from build123d import *

# Parameters (mm, degrees)
SKETCH1_W          = 25.4
SKETCH1_H          = 25.4
SKETCH1_W_2        = 19.05
SKETCH1_H_2        = 19.05
EXTRUDE1_DEPTH     = 558.8
SKETCH2_R          = 3.2639
CUT_EXTRUDE1_DEPTH = 26.4


with BuildPart() as part:
    # Sketch1 → Extrude1 (new body)
    with BuildSketch(Plane(origin=(0, 0, 0), x_dir=(0, 0, -1), z_dir=(1, 0, 0))):
        with Locations((12.7, 12.7)):
            Rectangle(SKETCH1_W, SKETCH1_H)
        with Locations((12.7, 12.7)):
            Rectangle(SKETCH1_W_2, SKETCH1_H_2, mode=Mode.SUBTRACT)
    extrude(amount=EXTRUDE1_DEPTH)

    # Sketch2 → Cut-Extrude1 (cut, through all)
    with BuildSketch(Plane(origin=(0, 25.4, 0), x_dir=(-1, 0, 0), z_dir=(0, 1, 0))):
        with Locations((-546.1, -12.7)):
            Circle(SKETCH2_R)
        with Locations((-368.3, -12.7)):
            Circle(SKETCH2_R)
        with Locations((-190.5, -12.7)):
            Circle(SKETCH2_R)
        with Locations((-12.7, -12.7)):
            Circle(SKETCH2_R)
    extrude(amount=-CUT_EXTRUDE1_DEPTH, mode=Mode.SUBTRACT)


solid = part.part
Model file for the job. Use its own axes, mm. A direction names the side the tool comes from. Coordinates: 2 decimals unless noted, no trailing zeros. Order: outer loops, then holes, each group sorted by start corner. A loop starts at its lowest first (then second) coordinate and runs counter-clockwise, first axis right, second up. Notation, with made-up numbers: M 83.5,21.5 L 122.5,21.5 A7 cw 122.5,25.5 Z; hole C -36,-2 d11. An arc over 180 degrees is marked long. Return JSON: item names as keys, results as strings.
1. Saw through at A-A (y = 16.75). Give the cut face in (x, z) (3 decimals), and give its area (3 significant figures).
Ans:
{"outline": "M 0,-25.4 L 558.8,-25.4 L 558.8,-22.225 L 0,-22.225 Z; M 0,-3.175 L 558.8,-3.175 L 558.8,0 L 0,0 Z", "area": "3,550 mm^2"}
2. Pull direction Z, two halves, no side cores. Call faces 1 (the face through (275, 13, -25.4)), 2 (the face through (275, 13, 0)), 3 (the face through (275, 13, -3.175)): +Z half, -Z half, draft (parallel to the pull), parting line (faces both ways), or undercut.
Ans:
{"face 1": "-Z half", "face 2": "+Z half", "face 3": "undercut"}
3. Flat gauge pin, fed straight in: pin 1 (5 mm diameter, centred on x = 368.3, z = -12.7, fed in from -Y). Where does the tip first touch, or does it go through?
Ans:
{"pin 1": "through"}
4. Drill centre lines: probe 1 along Y at (x, z) = (381.5, -13.75) (3 decimals); probe 2 along Z at (x, y) = (429, 21.25) (3 decimals); probe 3 along Z at (x, y) = (368.3, 1.85). Where is each one in solid material? Low to high.
Ans:
{"probe 1": "0 to 3.175, 22.225 to 25.4", "probe 2": "-25.4 to -22.225, -3.175 to 0", "probe 3": "-25.4 to -15.96, -9.44 to 0"}
5. Tool access for faces 4 (the face through (275, 0, -13)), 5 (the face through (275, 22.225, -13)): list every direction of +Z, -Z, +X, -X, +Y, -Y with a clear straight run to the whole face (end or side of a thin tool).
Ans:
{"face 4": "+Z, -Z, +X, -X, -Y", "face 5": "+X, -X"}
6. Saw through at B-B (x = 59). Give the cut face in (y, z) (3 decimals).
Ans:
{"outline": "M 0,-25.4 L 25.4,-25.4 L 25.4,0 L 0,0 Z; hole M 3.175,-22.225 L 22.225,-22.225 L 22.225,-3.175 L 3.175,-3.175 Z"}
